Work out the finished part from the listing and answer in its coordinate system (mm). Face numbers are marked on the shaded views. Give positions to 0.01 mm unless a question says otherwise; leave off trailing zeros. Use a Markdown table: item, result. Add a question column.
```python
from build123d import *

# Parameters (mm, degrees)
SKETCH1_W           = 52
SKETCH1_H           = 48
BOSS_EXTRUDE3_DEPTH = 2
SKETCH4_R           = 9
SKETCH4_R_2         = 7
SKETCH4_R_3         = 10
SKETCH4_R_4         = 8
SKETCH4_R_5         = 11
SKETCH4_R_6         = 12
BOSS_EXTRUDE4_DEPTH = 9
BOSS_EXTRUDE5_DEPTH = 9
SKETCH6_R           = 1
CUT_EXTRUDE2_DEPTH  = 6
SKETCH7_R           = 1
CUT_EXTRUDE3_DEPTH  = 6
FILLET1_R           = 5


with BuildPart() as part:
    # Sketch1 → Boss-Extrude3 (new body)
    with BuildSketch(Plane(origin=(0, 0, 0), x_dir=(1, 0, 0), z_dir=(0, 1, 0))):
        with Locations((-110.938964427, -50.099195195)):
            Rectangle(SKETCH1_W, SKETCH1_H)
    extrude(amount=BOSS_EXTRUDE3_DEPTH)

    # Sketch4 → Boss-Extrude4 (add)
    # profile 1 of 4: a face of its own
    with BuildSketch(Plane(origin=(0, 2, 0), x_dir=(1, 0, 0), z_dir=(0, 1, 0))):
        with Locations(Location((-125.938964427, -37.099195195, 0), (0, 0, 270))):
            Circle(SKETCH4_R)
        with Locations(Location((-125.938964427, -37.099195195, 0), (0, 0, 270))):
            Circle(SKETCH4_R_2, mode=Mode.SUBTRACT)
    # profile 2 of 4: a face of its own
    with BuildSketch(Plane(origin=(0, 2, 0), x_dir=(1, 0, 0), z_dir=(0, 1, 0))):
        with Locations(Location((-96.938964427, -38.099195195, 0), (0, 0, 270))):
            Circle(SKETCH4_R_3)
        with Locations(Location((-96.938964427, -38.099195195, 0), (0, 0, 270))):
            Circle(SKETCH4_R_4, mode=Mode.SUBTRACT)
    # profile 3 of 4: a face of its own
    with BuildSketch(Plane(origin=(0, 2, 0), x_dir=(1, 0, 0), z_dir=(0, 1, 0))):
        with Locations(Location((-97.938964427, -61.099195195, 0), (0, 0, 270))):
            Circle(SKETCH4_R_5)
        with Locations(Location((-97.938964427, -61.099195195, 0), (0, 0, 270))):
            Circle(SKETCH4_R, mode=Mode.SUBTRACT)
    # profile 4 of 4: a face of its own
    with BuildSketch(Plane(origin=(0, 2, 0), x_dir=(1, 0, 0), z_dir=(0, 1, 0))):
        with Locations(Location((-122.938964427, -60.099195195, 0), (0, 0, 270))):
            Circle(SKETCH4_R_6)
        with Locations(Location((-122.938964427, -60.099195195, 0), (0, 0, 270))):
            Circle(SKETCH4_R_3, mode=Mode.SUBTRACT)
    extrude(amount=BOSS_EXTRUDE4_DEPTH)

    # Sketch5 → Boss-Extrude5 (add)
    with BuildSketch(Plane(origin=(0, 2, 0), x_dir=(1, 0, 0), z_dir=(0, 1, 0))):
        with BuildLine():
            Line((-124.61601541, -59.599195195), (-122.938964427, -59.599195195))
            Line((-122.938964427, -59.599195195), (-121.261913444, -59.599195195))
            ThreePointArc((-121.261913444, -59.599195195), (-122.938964427, -58.349195195), (-124.61601541, -59.599195195))
        make_face()
        with BuildLine():
            Line((-121.261913444, -60.599195195), (-124.61601541, -60.599195195))
            ThreePointArc((-124.61601541, -60.599195195), (-122.938964427, -61.849195195), (-121.261913444, -60.599195195))
        make_face()
        with BuildLine():
            Line((-99.61601541, -60.599195195), (-97.938964427, -60.599195195))
            Line((-97.938964427, -60.599195195), (-96.261913444, -60.599195195))
            ThreePointArc((-96.261913444, -60.599195195), (-97.938964427, -59.349195195), (-99.61601541, -60.599195195))
        make_face()
        with BuildLine():
            Line((-96.261913444, -61.599195195), (-99.61601541, -61.599195195))
            ThreePointArc((-99.61601541, -61.599195195), (-97.938964427, -62.849195195), (-96.261913444, -61.599195195))
        make_face()
        with BuildLine():
            Line((-98.642636931, -37.699195195), (-96.938964427, -37.699195195))
            Line((-96.938964427, -37.699195195), (-95.235291923, -37.699195195))
            ThreePointArc((-95.235291923, -37.699195195), (-96.938964427, -36.349195195), (-98.642636931, -37.699195195))
        make_face()
        with BuildLine():
            Line((-95.235291923, -38.499195195), (-98.642636931, -38.499195195))
            ThreePointArc((-98.642636931, -38.499195195), (-96.938964427, -39.849195195), (-95.235291923, -38.499195195))
        make_face()
        with BuildLine():
            Line((-127.61601541, -36.599195195), (-125.938964427, -36.599195195))
            Line((-125.938964427, -36.599195195), (-124.261913444, -36.599195195))
            ThreePointArc((-124.261913444, -36.599195195), (-125.938964427, -35.349195195), (-127.61601541, -36.599195195))
        make_face()
        with BuildLine():
            Line((-124.261913444, -37.599195195), (-127.61601541, -37.599195195))
            ThreePointArc((-127.61601541, -37.599195195), (-125.938964427, -38.849195195), (-124.261913444, -37.599195195))
        make_face()
    extrude(amount=BOSS_EXTRUDE5_DEPTH)

    # Sketch6 → Cut-Extrude2 (cut)
    with BuildSketch(Plane.XY.offset(74.099195195)):
        with Locations((-97.938964427, 8)):
            Circle(SKETCH6_R)
        with Locations((-122.938964427, 8)):
            Circle(SKETCH6_R)
    extrude(amount=-CUT_EXTRUDE2_DEPTH, mode=Mode.SUBTRACT)

    # Sketch7 → Cut-Extrude3 (cut)
    with BuildSketch(Plane(origin=(0, 0, 26.099195195), x_dir=(-1, 0, 0), z_dir=(0, 0, -1))):
        with Locations(Location((96.938964427, 8, 0), (0, 0, 90))):
            Circle(SKETCH7_R)
        with Locations(Location((125.938964427, 8, 0), (0, 0, 90))):
            Circle(SKETCH7_R)
    extrude(amount=-CUT_EXTRUDE3_DEPTH, mode=Mode.SUBTRACT)

    # Fillet1
    fillet1_edges = [part.edges().sort_by_distance(p)[0] for p in [
        (-136.938964427, 1, 26.099195195),
        (-84.938964427, 1, 26.099195195),
        (-84.938964427, 1, 74.099195195),
        (-136.938964427, 1, 74.099195195),
    ]]
    fillet(fillet1_edges, radius=FILLET1_R)


solid = part.part
```
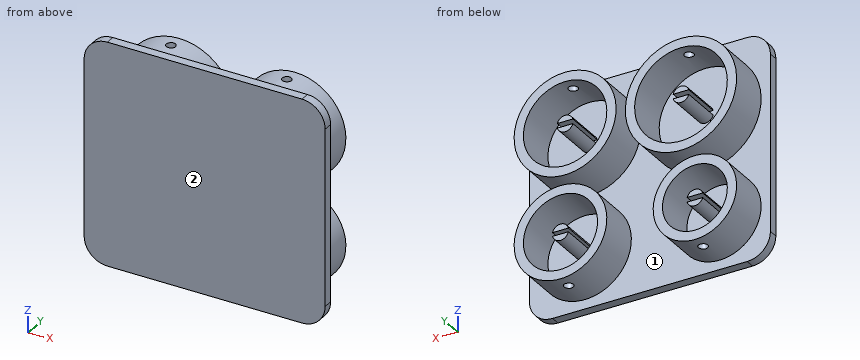
1) Straight lines are drawn through the part: line 1 (X direction, y = 5.5, z = 68.5); line 2 (X direction, y = 10.75, z = 43); line 3 (Z direction, x = -93.5, y = 10.25). For each, find the intervals that lie inside material, in ascending order.
2) Flat-ended cylindrical pins translate along their axes: pin 1 (1.7 mm diameter, centred on x = -123.5, y = 7.5, fed in from +Z); pin 2 (4 mm diameter, centred on x = -104.5, z = 64, fed in from +Y); pin 3 (3.5 mm diameter, centred on x = -122.5, y = 8.5, fed in from -Z); pin 4 (2 mm diameter, centred on y = 9.5, z = 55.5, fed in from -X). Find the tip coordinate at first contact, or state that the pin passes through.
3) The part is cut by section A-A, the plane y = 5.25. State how many separate pieces and enclosed holes the cut face has, then the cut area to 3 significant figures.
4) Determine the mould class of the marked faces 1 and 2 for opening direction Z: released by +Z, released by -Z, zero draft, split by the parting line, or undercut.
A:
| question | item | result |
|---|---|---|
| 1 | line 1 | -131.51 to -128.36, -117.51 to -114.37, -106.08 to -103.06, -92.82 to -89.8 |
| 1 | line 2 | -132.73 to -129.7, -122.17 to -119.14, -105.66 to -103.26, -90.62 to -88.22 |
| 1 | line 3 | 28.71 to 30.88, 45.32 to 47.49, 51.03 to 53.27, 68.93 to 71.16 |
| 2 | pin 1 | z = 72.1 |
| 2 | pin 2 | y = 11 |
| 2 | pin 3 | z = 28.26 |
| 2 | pin 4 | x = -134.39 |
| 3 | separate pieces | 12 |
| 3 | enclosed holes | 4 |
| 3 | area | 503 mm^2 |
| 4 | face 1 | undercut |
| 4 | face 2 | zero draft |
